Could you check a few things on this model? Use its own coordinates, in mm. A direction names the side the tool comes from. Round coordinates to 2 decimals unless told otherwise and drop trailing zeros. Order: outer loops, then holes, each group sorted by start corner. A loop starts at its lowest first (then second) coordinate and runs counter-clockwise, first axis right, second up. Notation, with made-up numbers: (-36.75, 32.5) - (-27.75, 32.5) arc R18 ccw to (-27.75, 47.5) - close; hole circle Ø11 at (55.25, 80.5). An arc over 180 degrees is marked (long way). Return JSON: item names as keys, results as strings. Group by question number.
from build123d import *

# Parameters (mm, degrees)
SKETCH_W     = 107
SKETCH_H     = 100
SKETCH_R     = 2.2
SKETCH_R_2   = 2.75
SKETCH_W_2   = 100
SKETCH_H_2   = 42
PAD_DEPTH    = 9
SKETCH001_W  = 45
SKETCH001_H  = 9
POCKET_DEPTH = 3
SKETCH004_W  = 15
SKETCH004_H  = 55
SKETCH004_R  = 3.25
PAD002_DEPTH = 3
FILLET_R     = 3


with BuildPart() as part:
    # Sketch → Pad (new body)
    with BuildSketch(Plane.XZ):
        with Locations((53.5, 30)):
            Rectangle(SKETCH_W, SKETCH_H)
        with Locations((7, 19.5)):
            Circle(SKETCH_R, mode=Mode.SUBTRACT)
        with Locations((100, 19.5)):
            Circle(SKETCH_R, mode=Mode.SUBTRACT)
        with Locations((7, 74.5)):
            Circle(SKETCH_R, mode=Mode.SUBTRACT)
        with Locations((100, 74.5)):
            Circle(SKETCH_R, mode=Mode.SUBTRACT)
        with Locations((10, -9)):
            Circle(SKETCH_R_2, mode=Mode.SUBTRACT)
        with Locations((93, -9)):
            Circle(SKETCH_R_2, mode=Mode.SUBTRACT)
        with Locations((53.5, 47)):
            Rectangle(SKETCH_W_2, SKETCH_H_2, mode=Mode.SUBTRACT)
    extrude(amount=PAD_DEPTH)

    # Sketch001 → Pocket (cut)
    with BuildSketch(Plane.XZ):
        with Locations((34.5, 75.5)):
            Rectangle(SKETCH001_W, SKETCH001_H)
    extrude(amount=POCKET_DEPTH, mode=Mode.SUBTRACT)

    # Sketch004 → Pad002 (join)
    with BuildSketch(Plane(origin=(0, -9, -10), x_dir=(1, 0, 0), z_dir=(0, -1, 0))):
        with Locations((-7.5, 17.5)):
            Rectangle(SKETCH004_W, SKETCH004_H)
        with Locations((-7.5, 20)):
            Circle(SKETCH004_R, mode=Mode.SUBTRACT)
        with Locations((-7.5, 35)):
            Circle(SKETCH004_R, mode=Mode.SUBTRACT)
    extrude(amount=-PAD002_DEPTH)

    # Fillet
    fillet_edges = [part.edges().sort_by_distance(p)[0] for p in [
        (0, -4.5, 80),
        (-15, -7.5, 35),
        (107, -4.5, 80),
    ]]
    fillet(fillet_edges, radius=FILLET_R)


solid = part.part
1) For faces 1 (the flat face through (34, -1, 71)), 2 (the flat face through (-11, -6, 8)), 3 (the flat face through (103.5, -4, 47)), which set-ups out of +Z, -Z, +X, -X, +Y, -Y let a thin tool reach every point of the face, with its end or its side?
2) I want a section at C-C, the plane z = 65. List the corners of the cut face in (x, y) for me.
3) I want a section at B-B, the plane x = 93. List the corners of the cut face in (y, z) for me, plus the area to 4 significant figures.
4) If I drill on line 1 along Z through (x, y) = (93, -5); line 2 along Z through (x, y) = (20, -7); line 3 along Z through (x, y) = (100, -6.5), over which ranges is the centre line in solid material (lowest first)? Write a range as from..to.
5) I want a section at D-D, the plane y = -7.5. Give the number of separate pieces and of enclosed holes in the cut face, plus the area to 3 significant figures.
6) We'd pull the mould along X, two halves only. Please class faces 4 (the flat face through (107, -4, 28)), 5 (the flat face through (53, -5, 80)), 6 (the cylindrical face through (-14.14, -7.48, 34.1)), 7 (the flat face through (53, -4, 26)): +X half, -X half, draft (parallel to the pull), parting line (faces both ways), or undercut.
7) Will these pins go through, and if not, where does the flat tip stop? pin 1 (2.5 mm diameter, centred on x = 26, z = 76, fed in from +Y); pin 2 (3.5 mm diameter, centred on y = -1.5, z = 75.5, fed in from -X).
8) I want a section at A-A, the plane z = -9. List the corners of the cut face in (x, y) for me, plus the area to 3 significant figures.
Outcome:
{
 "1": {"face 1": "+Z, +Y", "face 2": "+Z, -Z, -X, +Y", "face 3": "+Y, -Y"},
 "2": {"outline": "(0, -9) - (3.5, -9) - (3.5, 0) - (0, 0) - close; (103.5, -9) - (107, -9) - (107, 0) - (103.5, 0) - close"},
 "3": {"outline": "(-9, -20) - (0, -20) - (0, -11.75) - (-9, -11.75) - close; (-9, -6.25) - (0, -6.25) - (0, 26) - (-9, 26) - close; (-9, 68) - (0, 68) - (0, 80) - (-9, 80) - close", "area": "472.5 mm^2"},
 "4": {"line 1": "-20..-11.75, -6.25..26, 68..80", "line 2": "-20..26, 68..80", "line 3": "-20..17.3, 21.7..26, 68..72.3, 76.7..80"},
 "5": {"separate pieces": "1", "enclosed holes": "9", "area": "7,140 mm^2"},
 "6": {"face 4": "+X half", "face 5": "draft", "face 6": "-X half", "face 7": "undercut"},
 "7": {"pin 1": "y = -3", "pin 2": "x = 0"},
 "8": {"outline": "(-15, -9) - (7.25, -9) - (7.25, 0) - (0, 0) - (0, -6) - (-15, -6) - close; (12.75, -9) - (90.25, -9) - (90.25, 0) - (12.75, 0) - close; (95.75, -9) - (107, -9) - (107, 0) - (95.75, 0) - close", "area": "909 mm^2"}
}
